Input: dimensioned drawing with shaded views. Units: mm. Origin: part minimum x, y, z. Give positions to 0.01 mm unless a question says otherwise; leave off trailing zeros. Order: outer loops, then holes, each group sorted by start corner. A loop starts at its lowest first (then second) coordinate and runs counter-clockwise, first axis right, second up.
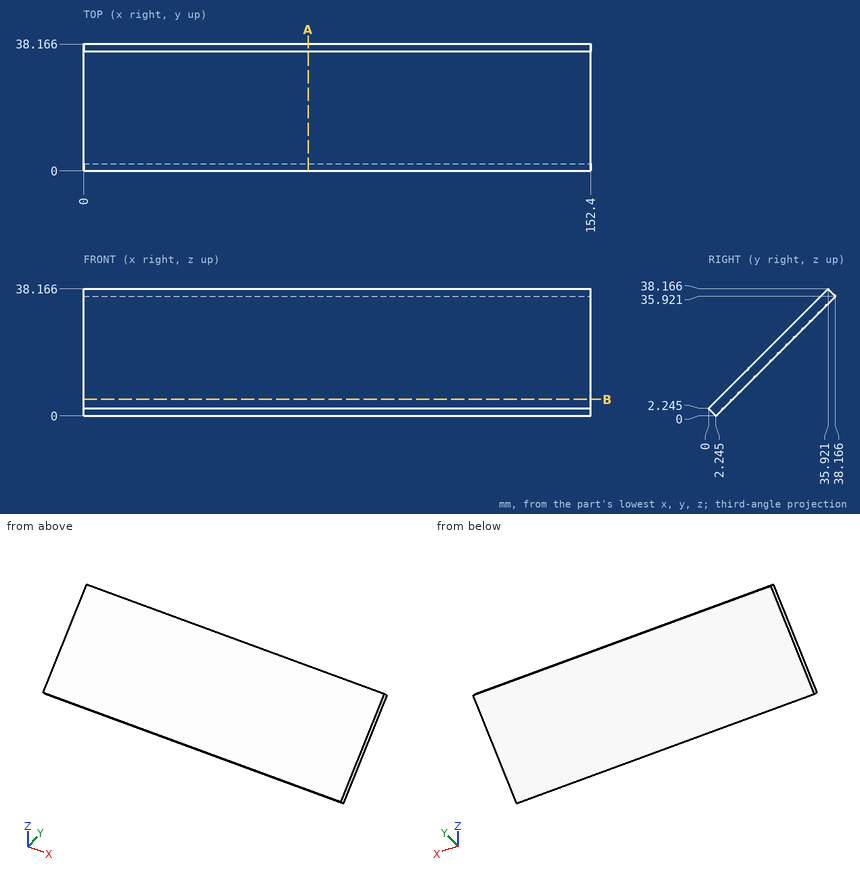
1) Section query A-A, the plane x = 67.5. Return the cut outline in (y, z) (3 decimals), and give its area (3 significant figures).
Report:
outline: (0, 2.245) - (2.245, 0) - (38.166, 35.921) - (35.921, 38.166) - close
area: 161 mm2
2) Pin query (flat end, axial travel): pin 1 (5 mm diameter, centred on x = 73.5, z = 19, fed in from -Y) (3 decimals); pin 2 (4 mm diameter, centred on x = 89, z = 31, fed in from -Y) (3 decimals); pin 3 (2 mm diameter, centred on x = 133, z = 32, fed in from -Y) (3 decimals). Return the tip coordinate at first contact, or that it passes through.
Report:
pin 1: stops at y = 14.255
pin 2: stops at y = 26.755
pin 3: stops at y = 28.755
3) Section query B-B, the plane z = 5. Return the cut outline in (x, y) (3 decimals).
Report:
outline: (0, 2.755) - (152.4, 2.755) - (152.4, 7.245) - (0, 7.245) - close
4) Material intervals for L1, parallel to Y at x = 98.5, z = 7.5 (1 decimal); L2, parallel to Y at x = 33, z = 3.5 (1 decimal); L3, parallel to Z at x = 37, y = 13.5 (1 decimal), sorted ascending.
Report:
L1: y = 5.3 to 9.7
L2: y = 1.3 to 5.7
L3: z = 11.3 to 15.7
